Autodesk Inventor part; units mm, degrees
ref_plane "YZ Plane" through (0, 0, 0) normal (1, 0, 0) x (0, 1, 0)
ref_plane "XZ Plane" through (0, 0, 0) normal (0, 1, 0) x (-1, 0, 0)
ref_plane "XY Plane" through (0, 0, 0) normal (0, 0, 1) x (1, 0, 0)
sketch "Sketch1" plane through (0, 0, 0) normal (0, 1, 0) x (-1, 0, 0)
  line L0 (235, 275) -> (-235, 275)
  line L1 (-235, 275) -> (-235, -275)
  line L2 (-235, -275) -> (235, -275)
  line L3 (235, -275) -> (235, 275)
  line L4 (235, 275) -> (-235, -275) construction
  line L5 (-235, 275) -> (235, -275) construction
  line L6 (232, 272) -> (-232, 272)
  line L7 (-232, 272) -> (-232, -272)
  line L8 (-232, -272) -> (232, -272)
  line L9 (232, -272) -> (232, 272)
  point P0 (0, 0)
  dimension "d0" = 470
  dimension "d1" = 550
  dimension "d2" = 3
extrude "Extrusion1" add sketch "Sketch1" along normal blind 3 contours L9 L8 L7 L6
extrude "Extrusion2" add sketch "Sketch1" along normal blind 690
fillet "Fillet1" radius 106 1 edges at (-232, 346.5, 272)
fillet "Fillet2" radius 148 1 edges at (-232, 346.5, -272)
fillet "Fillet3" radius 164 1 edges at (232, 346.5, 272)
fillet "Fillet4" radius 105 1 edges at (232, 346.5, -272)
fillet "Fillet5" radius 20 4 edges at (235, 345, 275) (235, 345, -275) (-235, 345, 275) (-235, 345, -275)
sketch "Sketch2" plane through (-215, 0, 275) normal (0, 0, 1) x (1, 0, 0)
  line L0 (0, 0) -> (0, 690)
  line L1 (0, 690) -> (430, 690)
  line L2 (0, 0) -> (430, 0)
  point P0 (215, 0)
  point P1 (215, 630)
  point P2 (215, 60)
  dimension "d19" = 215
  dimension "d20" = 60
  dimension "d21" = 215
  dimension "d22" = 60
hole "Hole1" at (0, 630, 275) at (0, 60, 275) direction (0, 0, -1) diameter 25.4 depth 26 tip angle 118
properties part number "Storage_tank"
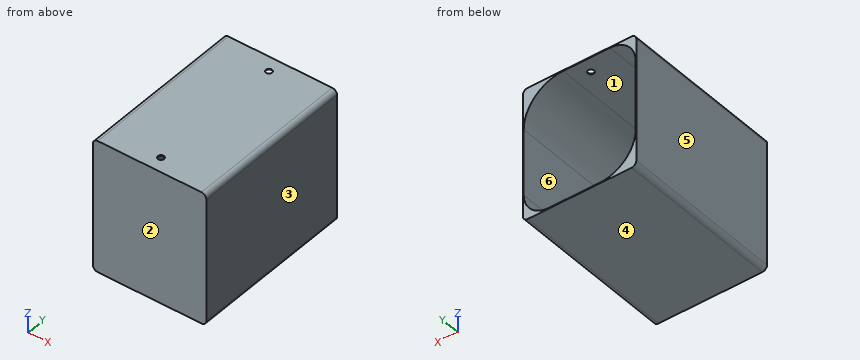
Model file for the job. Use its own axes, mm. Face numbers are marked on the shaded views. A direction names the side the tool comes from. Coordinates: 2 decimals unless noted, no trailing zeros. Order: outer loops, then holes, each group sorted by start corner. A loop starts at its lowest first (then second) coordinate and runs counter-clockwise, first axis right, second up. Notation, with made-up numbers: (-28.75, -4) -> (-24.75, -4) arc R20 cw to (-24.75, 15) -> close; hole circle Ø3 at (83, -9). An arc over 180 degrees is marked (long way). Return JSON: item names as keys, results as strings.
Item 1: Slice it at A-A (x = 0). Write the cut outline in (y, z), then the cut area to 3 significant figures.
Model answer:
{"outline": "(0, -275) -> (690, -275) -> (690, -272) -> (3, -272) -> (3, 272) -> (47.3, 272) -> (47.3, 275) -> (0, 275) -> close; (72.7, 272) -> (617.3, 272) -> (617.3, 275) -> (72.7, 275) -> close; (642.7, 272) -> (690, 272) -> (690, 275) -> (642.7, 275) -> close", "area": "5,620 mm²"}
Item 2: Slice it at B-B (y = 323). Write the cut outline in (x, z).
Model answer:
{"outline": "(-235, -255) arc R20 ccw to (-215, -275) -> (215, -275) arc R20 ccw to (235, -255) -> (235, 255) arc R20 ccw to (215, 275) -> (-215, 275) arc R20 ccw to (-235, 255) -> close; hole (-232, -124) arc R148 ccw to (-84, -272) -> (127, -272) arc R105 ccw to (232, -167) -> (232, 108) arc R164 ccw to (68, 272) -> (-126, 272) arc R106 ccw to (-232, 166) -> close"}
Item 3: Mould opens along X. For the marked faces 3, 4, 5 and 6 say: pulls with the +X half, pulls with the -X half, needs draft (parallel to the pull), parting line crosses it, or undercut.
Model answer:
{"face 3": "pulls with the +X half", "face 4": "needs draft", "face 5": "pulls with the -X half", "face 6": "undercut"}
Item 4: Wall check: line 1 along Y through (x, z) = (0, 273); line 2 along Z through (x, y) = (67.5, 133); line 3 along X through (y, z) = (129, 90). Give the ranges that are in metal, low to high. Write a range as from..to.
Model answer:
{"line 1": "y = 0..47.3, 72.7..617.3, 642.7..690", "line 2": "z = -275..-272, 272..275", "line 3": "x = -235..-232, 232..235"}
Item 5: 3-axis set-ups, long thin cutter, end or side, ignore diameter. For the marked faces 1 and 2: which of +Z, -Z, +X, -X, +Y, -Y reach the whole face in a straight line?
Model answer:
{"face 1": "+Y", "face 2": "+Z, -Z, +X, -X, -Y"}
Item 6: Slice it at C-C (z = 14.5). Write the cut outline in (x, y).
Model answer:
{"outline": "(-235, 0) -> (235, 0) -> (235, 690) -> (232, 690) -> (232, 3) -> (-232, 3) -> (-232, 690) -> (-235, 690) -> close"}
Item 7: Slice it at D-D (y = 60). Write the cut outline in (x, z).
Model answer:
{"outline": "(-235, -255) arc R20 ccw to (-215, -275) -> (215, -275) arc R20 ccw to (235, -255) -> (235, 255) arc R20 ccw to (215, 275) -> (12.7, 275) -> (12.7, 272) -> (68, 272) arc R164 cw to (232, 108) -> (232, -167) arc R105 cw to (127, -272) -> (-84, -272) arc R148 cw to (-232, -124) -> (-232, 166) arc R106 cw to (-126, 272) -> (-12.7, 272) -> (-12.7, 275) -> (-215, 275) arc R20 ccw to (-235, 255) -> close"}
Item 8: Pin check, flat tips, straight feed: P1, Ø1, axis at x = 10, z = 26, coming from the +Y side; P2, Ø15, axis at x = 0, y = 630, coming from the +Z side. Stop position of each tip, or through.
Model answer:
{"P1": "stops at y = 3", "P2": "stops at z = -272"}
